The listing builds one solid part. Answer for the finished solid, in the listing's coordinates (mm). Face numbers are marked on the shaded views. A direction names the side the tool comes from. Round coordinates to 2 decimals unless told otherwise and drop trailing zeros. Order: outer loops, then holes, each group sorted by start corner. A loop starts at its lowest first (then second) coordinate and runs counter-clockwise, first axis right, second up. Notation, with made-up numbers: (53, 73) -> (93, 73) arc R27 ccw to (93, 94) -> close; hole circle Ø4 at (11, 57). An arc over 180 degrees is marked (long way). Return JSON: item names as keys, results as strings. Group by question number.
(1) The part is cut by section B-B (y = 13). Determine the outline of the cut face in (x, z) (3 decimals), plus the area to 3 significant figures.
(2) Which of the six approach directions +Z, -Z, +X, -X, +Y, -Y give full straight-line access (tool end or side, diameter ignored) to the marked faces 1, 2 and 3?
(3) Determine the mould class of the marked faces 4, 5 and 6 for opening direction X: +X half, -X half, draft (parallel to the pull), parting line (faces both ways), or undercut.
(4) Consider line 1 (X direction, y = 12, z = 11.5); line 2 (X direction, y = 7.5, z = 17); line 3 (Z direction, x = -47, y = 3). Determine where each line is inside the solid, lowest interval first. Write a range as [from, to].
(5) The part is cut by section C-C (z = 29). Determine the outline of the cut face in (x, y).
(6) The part is cut by section D-D (y = -1). Determine the outline of the cut face in (x, z) (3 decimals), plus the area to 3 significant figures.
(7) The part is cut by section A-A (z = 6.5). Determine the outline of the cut face in (x, y) (3 decimals), plus the area to 3 significant figures.
(8) Each of these flat-tipped pins is pushed along its axis until it touches: pin 1 (4 mm diameter, centred on x = -23.5, y = 7.5, fed in from +Z); pin 2 (16.5 mm diameter, centred on x = 10, y = 4.5, fed in from +Z); pin 3 (1.5 mm diameter, centred on x = -58.5, y = 6.5, fed in from +Z). Where does it stop, or does it pass through?
from build123d import *

# Parameters (mm, degrees)
F0_W     = 8.89
F0_H     = 25.618968
F1_DEPTH = 19.05
F2_R     = 5.08
F4_D     = 6.35


with BuildPart() as f1:
    # F0 (on Front) → F1 (new body, symmetric)
    with BuildSketch(Plane.XZ):
        Polygon((-70.550688, 2.037292), (-31.114999, 2.037292), (-31.114999, 10.927292), (-40.004999, 10.927292), (-70.550688, 10.927292), align=None)
        Polygon((0.555625, 10.927292), (-8.334375, 10.927292), (-8.334375, 2.037292), (24.262293, 2.037292), (24.262293, 10.927292), (15.372293, 10.927292), align=None)
        with BuildLine():
            Line((-40.004999, 10.927292), (-31.114999, 10.927292))
            ThreePointArc((-31.114999, 10.927292), (-19.724687, 22.317604), (-8.334375, 10.927292))
            Line((-8.334375, 10.927292), (0.555625, 10.927292))
            ThreePointArc((0.555625, 10.927292), (-19.724687, 31.207604), (-40.004999, 10.927292))
        make_face()
        with Locations((19.817293, 23.736776)):
            Rectangle(F0_W, F0_H)
    extrude(amount=F1_DEPTH, both=True)

    # F2
    f2_edges = [f1.edges().sort_by_distance(p)[0] for p in [
        (-70.550688, -19.05, 6.482292),
        (-70.550688, 19.05, 6.482292),
        (19.817293, -19.05, 36.54626),
        (19.817293, 19.05, 36.54626),
    ]]
    fillet(f2_edges, radius=F2_R)

    # F4 (through all)
    with Locations(Plane.XY.offset(10.927292)):
        with Locations((-58.325827, 13.97), (-58.325827, -13.97)):
            Hole(F4_D / 2)


solid = f1.part
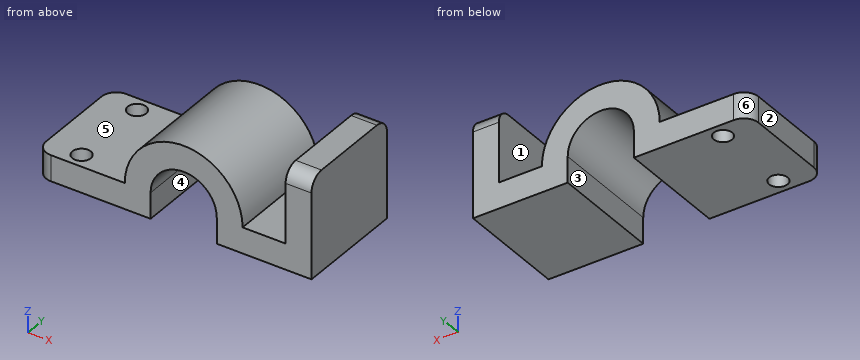
Answer below:
{
 "1": {"outline": "(-70.551, 2.037) -> (-61.349, 2.037) -> (-61.349, 10.927) -> (-70.551, 10.927) -> close; (-55.303, 2.037) -> (-31.115, 2.037) -> (-31.115, 10.927) arc R11.39 cw to (-8.334, 10.927) -> (-8.334, 2.037) -> (24.262, 2.037) -> (24.262, 36.546) -> (15.372, 36.546) -> (15.372, 10.927) -> (0.556, 10.927) arc R20.28 ccw to (-40.005, 10.927) -> (-55.303, 10.927) -> close", "area": "1,260 mm²"},
 "2": {"face 1": "+Z, +Y, -Y", "face 2": "+Z, -Z, -X, +Y, -Y", "face 3": "-Z, +Y, -Y"},
 "3": {"face 4": "undercut", "face 5": "draft", "face 6": "-X half"},
 "4": {"line 1": "x = [-40, -31.1], [-8.35, 0.55], [15.37, 24.26]", "line 2": "x = [-39.07, -29.36], [-10.09, -0.37], [15.37, 24.26]", "line 3": "z = [2.04, 10.93]"},
 "5": {"outline": "(-28.93, -19.05) -> (-10.52, -19.05) -> (-10.52, 19.05) -> (-28.93, 19.05) -> close; (15.37, -19.05) -> (24.26, -19.05) -> (24.26, 19.05) -> (15.37, 19.05) -> close"},
 "6": {"outline": "(-70.551, 2.037) -> (-31.115, 2.037) -> (-31.115, 10.927) arc R11.39 cw to (-8.334, 10.927) -> (-8.334, 2.037) -> (24.262, 2.037) -> (24.262, 36.546) -> (15.372, 36.546) -> (15.372, 10.927) -> (0.556, 10.927) arc R20.28 ccw to (-40.005, 10.927) -> (-70.551, 10.927) -> close", "area": "1,310 mm²"},
 "7": {"outline": "(-70.551, -13.97) arc R5.08 ccw to (-65.471, -19.05) -> (-31.115, -19.05) -> (-31.115, 19.05) -> (-65.471, 19.05) arc R5.08 ccw to (-70.551, 13.97) -> close; (-8.334, -19.05) -> (24.262, -19.05) -> (24.262, 19.05) -> (-8.334, 19.05) -> close; hole circle Ø6.35 at (-58.326, -13.97); hole circle Ø6.35 at (-58.326, 13.97)", "area": "2,670 mm²"},
 "8": {"pin 1": "stops at z = 31.13", "pin 2": "stops at z = 36.55", "pin 3": "stops at z = 10.93"}
}
